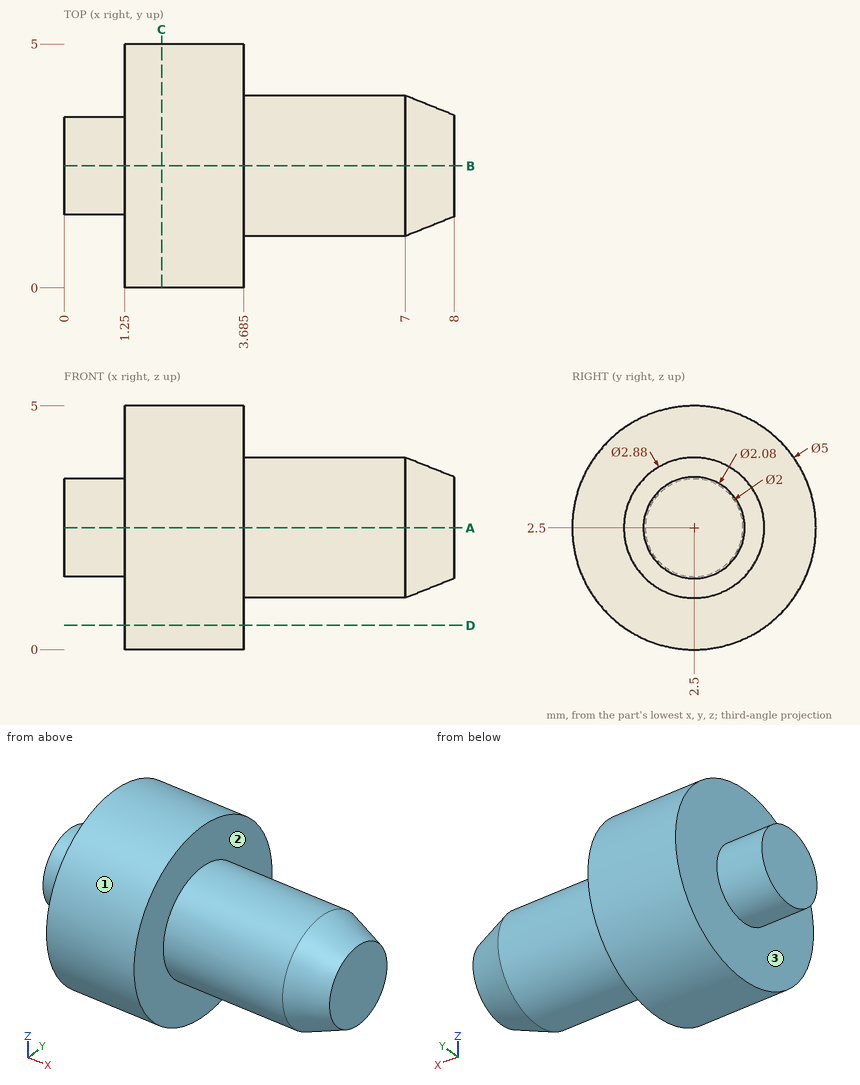
Print and shaded views of the part. All mm, measured from the part's lowest x, y and z. A direction names the side the tool comes from. Coordinates: 2 decimals unless noted, no trailing zeros. Loops run counter-clockwise (first coordinate to the right, second up) from the corner with the lowest first, then second, coordinate; pieces in that order, holes last. Notation, with made-up numbers: (76.5, 29.25) -> (106.5, 29.25) arc R21 ccw to (106.5, 49.25) -> close; hole circle Ø3 at (2.25, 9.25). An arc over 180 degrees is marked (long way). Use a Markdown table: item, result. Add a question column.
Item 1: Band-saw the part on D-D on z = 0.5. Write the cut outline in (x, y) (3 decimals), plus the area to 4 significant figures.
Item 2: Which spindle directions (+Z, -Z, +X, -X, +Y, -Y) get a long thin tool onto all of the face, cutting with end or side? Do the marked faces 1, 2 and 3. Say none if no direction does.
Item 3: Band-saw the part on C-C on x = 2. Write the cut outline in (y, z), plus the area to 3 significant figures.
Item 4: Band-saw the part on A-A on z = 2.5. Write the cut outline in (x, y) (3 decimals), plus the area to 3 significant figures.
Item 5: Probe probe 1 along X at (y, z) = (2.15, 0.3) (3 decimals); probe 2 along X at (y, z) = (1.6, 3.45); probe 3 along Y at (x, z) = (2.5, 0.3). List the from-to ranges inside material, lowest first.
Item 6: Flat gauge pins, fed straight in: P1, Ø3, axis at x = 2.5, z = 1.5, coming from the +Y side; P2, Ø1, axis at y = 1, z = 4, coming from the +X side (3 decimals); P3, Ø1, axis at x = 7, y = 2, coming from the -Z side; P4, Ø2, axis at x = 2.5, z = 1, coming from the +Y side. Where does each tip first touch, or does it go through?
Geometry says:
| question | item | result |
|---|---|---|
| 1 | outline | (1.25, 1) -> (3.685, 1) -> (3.685, 4) -> (1.25, 4) -> close |
| 1 | area | 7.305 mm² |
| 2 | face 1 | +X, -X |
| 2 | face 2 | +X |
| 2 | face 3 | -X |
| 3 | outline | circle Ø5 at (2.5, 2.5) |
| 3 | area | 19.6 mm² |
| 4 | outline | (0, 1.5) -> (1.25, 1.5) -> (1.25, 0) -> (3.685, 0) -> (3.685, 1.06) -> (7, 1.06) -> (8, 1.46) -> (8, 3.54) -> (7, 3.94) -> (3.685, 3.94) -> (3.685, 5) -> (1.25, 5) -> (1.25, 3.5) -> (0, 3.5) -> close |
| 4 | area | 26.7 mm² |
| 5 | probe 1 | 1.25 to 3.685 |
| 5 | probe 2 | 1.25 to 7.33 |
| 5 | probe 3 | 1.31 to 3.69 |
| 6 | P1 | y = 5 |
| 6 | P2 | x = 3.685 |
| 6 | P3 | z = 1.06 |
| 6 | P4 | y = 4.95 |
